```python
from build123d import *

# Parameters (mm, degrees)
BOSS_EXTRUDE1_DEPTH     = 6
SKETCH2_R               = 23
BOSS_EXTRUDE2_DEPTH     = 4
SKETCH4_R               = 45
BOSS_EXTRUDE3_DEPTH     = 6
SKETCH5_R               = 40
CUT_EXTRUDE1_DEPTH      = 6
SKETCH6_R               = 19
BOSS_EXTRUDE4_DEPTH     = 6
SKETCH7_R               = 14
CUT_EXTRUDE2_DEPTH      = 8
SKETCH8_R               = 7
CUT_EXTRUDE3_DEPTH      = 83.524743764
CUT_EXTRUDE4_DEPTH      = 82.574097196
CUT_EXTRUDE4_DEPTH_BACK = 82.574097196
SKETCH9_R               = 3.5
FILLET1_R               = 5
FILLET2_R               = 4
FILLET3_R               = 2
CHAMFER1_SIZE           = 1


with BuildPart() as part:
    # Sketch1 → Boss-Extrude1 (new body)
    with BuildSketch(Plane.XY):
        Polygon((0, 61.199128534), (-53, 30.599564267), (-53, -30.599564267), (0, -61.199128534), (53, -30.599564267), (53, 30.599564267), align=None)
    extrude(amount=-BOSS_EXTRUDE1_DEPTH)

    # Sketch2 → Boss-Extrude2 (add)
    with BuildSketch(Plane(origin=(0, 0, -6), x_dir=(-1, 0, 0), z_dir=(0, 0, -1))):
        Circle(SKETCH2_R)
    extrude(amount=BOSS_EXTRUDE2_DEPTH)

    # Sketch4 → Boss-Extrude3 (add)
    with BuildSketch(Plane.XY):
        Circle(SKETCH4_R)
    extrude(amount=BOSS_EXTRUDE3_DEPTH)

    # Sketch5 → Cut-Extrude1 (cut)
    with BuildSketch(Plane.XY.offset(6)):
        Circle(SKETCH5_R)
    extrude(amount=-CUT_EXTRUDE1_DEPTH, mode=Mode.SUBTRACT)

    # Sketch6 → Boss-Extrude4 (add)
    with BuildSketch(Plane.XY):
        Circle(SKETCH6_R)
    extrude(amount=BOSS_EXTRUDE4_DEPTH)

    # Sketch7 → Cut-Extrude2 (cut)
    with BuildSketch(Plane.XY.offset(6)):
        Circle(SKETCH7_R)
    extrude(amount=-CUT_EXTRUDE2_DEPTH, mode=Mode.SUBTRACT)

    # Sketch8 → Cut-Extrude3 (cut, through all)
    with BuildSketch(Plane(origin=(0, 0, -10), x_dir=(-1, 0, 0), z_dir=(0, 0, -1))):
        Circle(SKETCH8_R)
    extrude(amount=-CUT_EXTRUDE3_DEPTH, mode=Mode.SUBTRACT)

    # Sketch9 → Cut-Extrude4 (cut, two sides: drawn at the far end of the back side and taken through both)
    with BuildSketch(Plane.XY.offset(-CUT_EXTRUDE4_DEPTH_BACK)):
        with Locations((0, 51)):
            Circle(SKETCH9_R)
        with Locations((44.167295593, 25.5)):
            Circle(SKETCH9_R)
        with Locations((44.167295593, -25.5)):
            Circle(SKETCH9_R)
        with Locations((0, -51)):
            Circle(SKETCH9_R)
        with Locations((-44.167295593, -25.5)):
            Circle(SKETCH9_R)
        with Locations((-44.167295593, 25.5)):
            Circle(SKETCH9_R)
    extrude(amount=CUT_EXTRUDE4_DEPTH + CUT_EXTRUDE4_DEPTH_BACK, mode=Mode.SUBTRACT)

    # Fillet1
    fillet1_edges = [part.edges().sort_by_distance(p)[0] for p in [
        (53, 30.599564267, -3),
        (53, -30.599564267, -3),
        (0, -61.199128534, -3),
        (-53, -30.599564267, -3),
        (-53, 30.599564267, -3),
        (0, 61.199128534, -3),
    ]]
    fillet(fillet1_edges, radius=FILLET1_R)

    # Fillet2
    fillet2_edges = [part.edges().sort_by_distance(p)[0] for p in [
        (23, 0, -6),
    ]]
    fillet(fillet2_edges, radius=FILLET2_R - 0.0001)  # a hair under: the kernel refuses the full size

    # Fillet3
    fillet3_edges = [part.edges().sort_by_distance(p)[0] for p in [
        (-40, 0, 0),
        (-19, 0, 0),
        (26.5, 45.899346401, -6),
        (-26.5, 45.899346401, -6),
        (53, 0, -6),
        (26.5, -45.899346401, -6),
        (-26.5, -45.899346401, -6),
        (-53, 0, -6),
        (-52.330127019, 30.212812921, -6),
        (52.330127019, 30.212812921, -6),
        (52.330127019, -30.212812921, -6),
        (0, -60.425625842, -6),
        (-52.330127019, -30.212812921, -6),
        (0, 60.425625842, -6),
    ]]
    fillet(fillet3_edges, radius=FILLET3_R)

    # Chamfer1
    chamfer1_edges = [part.edges().sort_by_distance(p)[0] for p in [
        (-45, 0, 6),
        (-19, 0, 6),
    ]]
    chamfer(chamfer1_edges, length=CHAMFER1_SIZE)


solid = part.part
```
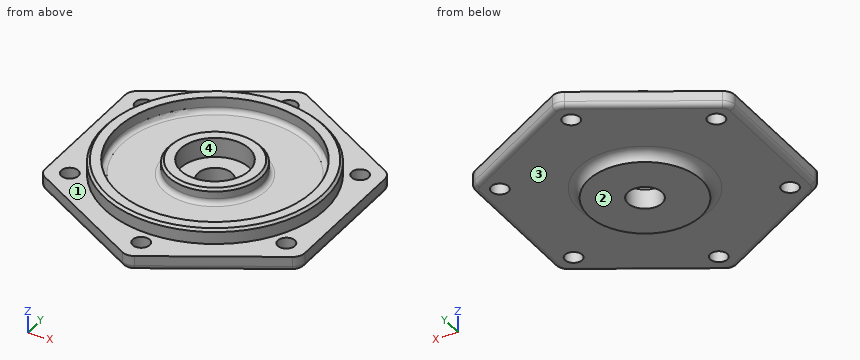
The model under review builds one solid part; all positions refer to its coordinate system, in mm. Face numbers are marked on the shaded views. A direction names the side the tool comes from. Round coordinates to 2 decimals unless told otherwise and drop trailing zeros. Put each result on its own line as item: value.
Q1. For pin 1 (4 mm diameter, centred on y = 45.5, z = 0, fed in from -X); pin 2 (9 mm diameter, centred on x = -44.17, y = 25.5, fed in from -Z); pin 3 (5 mm diameter, centred on x = 36.5, z = -4.5, fed in from -Y), all flat-tipped, find the tip position at first contact; note any pin that passes through.
Result set:
pin 1: stops at x = -30.66
pin 2: stops at z = -6
pin 3: stops at y = -41.55
Q2. Machinability: for the marked faces 1 and 2, which of the approach directions +Z, -Z, +X, -X, +Y, -Y give a long, thin tool a straight path to every point of the face, cutting with its end or side? Answer none if there is none.
Result set:
face 1: +Z
face 2: -Z, +X, -X, +Y, -Y
Q3. Consider section A-A, the plane x = 0. Count the separate pieces of the cut face and the enclosed holes in it, then the cut area to 3 significant figures.
Result set:
separate pieces: 4
enclosed holes: 0
area: 784 mm²
Q4. To check wall thickness, follow L1, parallel to Y at x = 0, z = -3.5; L2, parallel to X at y = -25.5, z = -3.5; L3, parallel to Y at x = 0, z = 3.5. State the ranges of each line that lie inside material, in increasing order.
Result set:
L1: y = -60.43 to -54.5, -47.5 to -7, 7 to 47.5, 54.5 to 60.43
L2: x = -53 to -47.67, -40.67 to 40.67, 47.67 to 53
L3: y = -45 to -40, -19 to -14, 14 to 19, 40 to 45
Q5. Mouldability with a two-part tool opening along Y and no side actions: class the marked faces 3 and 4 as released by +Y, released by -Y, zero draft, split by the parting line, or undercut.
Result set:
face 3: zero draft
face 4: undercut
